```python
from build123d import *

# Parameters (mm, degrees)
PAD_DEPTH       = 5
POCKET_DEPTH    = 4
SKETCH005_R     = 15
PAD001_DEPTH    = 4
FILLET_R        = 1
FILLET001_R     = 0.5
SKETCH006_R     = 14
POCKET001_DEPTH = 5.001
FILLET002_R     = 1
FILLET003_R     = 1
FILLET004_R     = 1
FILLET005_R     = 1
FILLET006_R     = 1
FILLET007_R     = 1
FILLET008_R     = 1


with BuildPart() as part:
    # Sketch001 → Pad (new body)
    with BuildSketch(Plane.XY):
        with BuildLine():
            Line((29.31354, 7.607129), (11.31354, 7.607129))
            ThreePointArc((11.31354, 7.607129), (-23, 0), (11.31354, -7.607129))
            Line((11.31354, -7.607129), (29.31354, -7.607129))
            Line((29.31354, 7.607129), (29.31354, -7.607129))
        make_face()
    extrude(amount=PAD_DEPTH)

    # Sketch004 → Pocket (cut)
    with BuildSketch(Plane.XY):
        with BuildLine():
            Line((28.648583, 6.642429), (10.648583, 6.642429))
            ThreePointArc((10.648583, 6.642429), (-22, 0), (10.648583, -6.642429))
            Line((10.648583, -6.642429), (28.648583, -6.642429))
            Line((28.648583, -1), (28.648583, -6.642429))
            Line((32.648583, -1), (28.648583, -1))
            Line((32.648583, 1), (32.648583, -1))
            Line((28.648583, 1), (32.648583, 1))
            Line((28.648583, 6.642429), (28.648583, 1))
        make_face()
    extrude(amount=POCKET_DEPTH, mode=Mode.SUBTRACT)

    # Sketch005 → Pad001 (join)
    with BuildSketch(Plane.XY.offset(1)):
        with Locations((-5, 0)):
            Circle(SKETCH005_R)
    extrude(amount=PAD001_DEPTH)

    # Fillet
    fillet_edges = [part.edges().sort_by_distance(p)[0] for p in [
        (-23, 0, 5),
    ]]
    fillet(fillet_edges, radius=FILLET_R)

    # Fillet001
    fillet001_edges = [part.edges().sort_by_distance(p)[0] for p in [
        (-23, 0, 0),
    ]]
    fillet(fillet001_edges, radius=FILLET001_R)

    # Sketch006 → Pocket001 (cut, through all)
    with BuildSketch(Plane.XY):
        with Locations((-5, 0)):
            Circle(SKETCH006_R)
    extrude(amount=POCKET001_DEPTH, mode=Mode.SUBTRACT)

    # Fillet002
    fillet002_edges = [part.edges().sort_by_distance(p)[0] for p in [
        (-19, 0, 5),
    ]]
    fillet(fillet002_edges, radius=FILLET002_R)

    # Fillet003
    fillet003_edges = [part.edges().sort_by_distance(p)[0] for p in [
        (28.981061, 1, 0),
    ]]
    fillet(fillet003_edges, radius=FILLET003_R)

    # Fillet004
    fillet004_edges = [part.edges().sort_by_distance(p)[0] for p in [
        (28.981061, -1, 0),
    ]]
    fillet(fillet004_edges, radius=FILLET004_R)

    # Fillet005
    fillet005_edges = [part.edges().sort_by_distance(p)[0] for p in [
        (29.31354, 7.607129, 2.5),
    ]]
    fillet(fillet005_edges, radius=FILLET005_R)

    # Fillet006
    fillet006_edges = [part.edges().sort_by_distance(p)[0] for p in [
        (29.31354, -7.607129, 2.5),
    ]]
    fillet(fillet006_edges, radius=FILLET006_R)

    # Fillet007
    fillet007_edges = [part.edges().sort_by_distance(p)[0] for p in [
        (10.648583, 6.642429, 2),
    ]]
    fillet(fillet007_edges, radius=FILLET007_R)

    # Fillet008
    fillet008_edges = [part.edges().sort_by_distance(p)[0] for p in [
        (10.648583, -6.642429, 2),
    ]]
    fillet(fillet008_edges, radius=FILLET008_R)


solid = part.part
```
Geometry check sheet. Reference: the model listing, model coordinates, mm. A direction names the side the tool comes from. Coordinates: 2 decimals unless noted, no trailing zeros. Order: outer loops, then holes, each group sorted by start corner. A loop starts at its lowest first (then second) coordinate and runs counter-clockwise, first axis right, second up. Notation, with made-up numbers: M 85.5,56 L 136.5,56 A18 ccw 136.5,77 Z; hole C 28.5,-25 d7. An arc over 180 degrees is marked long. One line per question, with ' | ' between items. Start each with the question number.
Item 1: Cross-section at A-A on y = 0. Enter the section's corners in (x, z), then the cut area to 3 significant figures.
Item 2: Cross-section at C-C on x = 14.5. Enter the section's corners in (y, z), then the cut area to 3 significant figures.
Item 3: Draft check along X on faces 1 (the cylindrical face through (29.028, -7.306, 2.535)), 2 (the cylindrical face through (-21.988, 0.643, 1.972)), 3 (the cylindrical face through (-18.986, 0.616, 2.479)), 4 (the flat face through (19, 7.607, 2)). Enter one of: pulls with the +X half, pulls with the -X half, needs draft (parallel to the pull), parting line crosses it, or undercut.
Item 4: Cross-section at B-B on z = 2.55. Enter the section's corners in (x, y), then the cut area to 3 significant figures.
Item 5: Material ranges on L1, parallel to X at y = 0, z = 1.25; L2, parallel to Y at x = -4.5, z = 1.9; L3, parallel to Y at x = 18, z = 2.55, recorded low to high. Write a range as [from, to].
Item 6: Set-up check for faces 5 (the cylindrical face through (29.028, 7.306, 2.535)), 6 (the flat face through (11, 0, 4)), 7 (the cylindrical face through (28.976, -1.301, 0.285)): record each of +Z, -Z, +X, -X, +Y, -Y from which the full face is reachable in a straight line by a thin tool's end or side.
Item 7: Gauge pin test, flat ends, axial feed: pin 1 (3 mm diameter, centred on x = 13.5, z = 2.5, fed in from +Y); pin 2 (10 mm diameter, centred on x = 16, y = 1.5, fed in from -Z); pin 3 (1.5 mm diameter, centred on x = 15, z = 2, fed in from -Y). Record the tip position at first contact, or that the pin passes through.
Findings:
1) outline: M -23,0.5 A0.5 ccw -22.5,0 L -22,0 L -22,4 L -20,4 L -20,1 L -19,1 L -19,4 A1 ccw -20,5 L -22,5 A1 ccw -23,4 Z; M 9,1 L 10,1 L 10,4 L 29.31,4 L 29.31,5 L 10,5 A1 ccw 9,4 Z | area: 33.6 mm²
2) outline: M -7.61,0 L -6.64,0 L -6.64,4 L 6.64,4 L 6.64,0 L 7.61,0 L 7.61,5 L -7.61,5 Z | area: 22.9 mm²
3) face 1: pulls with the +X half | face 2: undercut | face 3: undercut | face 4: needs draft
4) outline: C -5,0 d30; M 10.39,-7.22 A17 cw long 10.39,7.22 A1 ccw 11.3,6.64 L 28.65,6.64 L 28.65,1 L 29.31,1 L 29.31,6.61 A1 ccw 28.31,7.61 L 11.31,7.61 A18 ccw long 11.31,-7.61 L 28.31,-7.61 A1 ccw 29.31,-6.61 L 29.31,-1 L 28.65,-1 L 28.65,-6.64 L 11.3,-6.64 A1 ccw Z; hole C -5,0 d28 | area: 229 mm²
5) L1: x = [-23, -22], [-20, -19], [9, 10] | L2: y = [-17.99, -16.99], [-14.99, -13.99], [13.99, 14.99], [16.99, 17.99] | L3: y = [-7.61, -6.64], [6.64, 7.61]
6) face 5: +Z, -Z, +X, +Y | face 6: -Z | face 7: -Z, +X
7) pin 1: stops at y = 7.61 | pin 2: stops at z = 4 | pin 3: stops at y = -7.61
